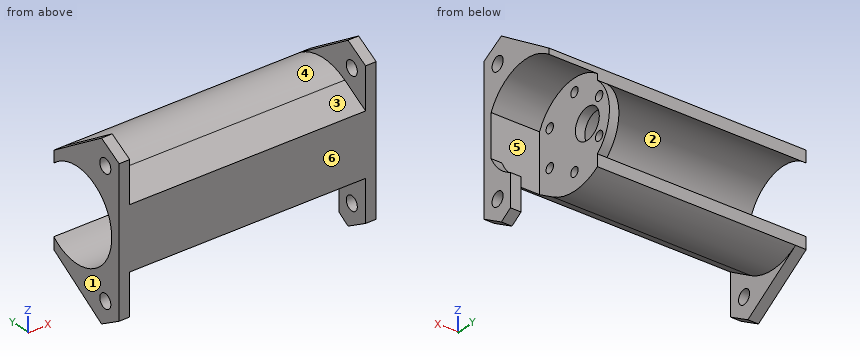
from build123d import *

# Parameters (mm, degrees)
SKETCH1_R           = 3
BOSS_EXTRUDE1_DEPTH = 54.5
CUT_EXTRUDE1_DEPTH  = 50
BOSS_EXTRUDE2_START = 34
SKETCH3_R           = 19
SKETCH3_R_2         = 6.5
SKETCH3_R_3         = 2
BOSS_EXTRUDE2_DEPTH = 4
CUT_EXTRUDE2_DEPTH  = 20.5
SKETCH5_W           = 31.652494028
SKETCH5_H           = 22.199486155
CUT_EXTRUDE3_DEPTH  = 16


# Read off the part's stored shape, not the designer's step: Cut-Extrude2
with BuildPart() as part:
    # Sketch1 → Boss-Extrude1 (new, symmetric)
    with BuildSketch(Plane(origin=(0, 0, 0), x_dir=(0, 0, -1), z_dir=(1, 0, 0))):
        with BuildLine():
            Line((26.267851073, -23), (0, -23))
            Line((0, -23), (-26.267851073, -23))
            Line((-26.267851073, -23), (-30.597978092, -23))
            Line((-30.597978092, -23), (-36.109878886, -13.453107779))
            Line((-36.109878886, -13.453107779), (-19.306734576, 12.5))
            Line((-19.306734576, 12.5), (-14.309088021, 12.5))
            ThreePointArc((-14.309088021, 12.5), (0, -19), (14.309088021, 12.5))
            Line((14.309088021, 12.5), (19.306734576, 12.5))
            Line((19.306734576, 12.5), (36.109878886, -13.453107779))
            Line((36.109878886, -13.453107779), (30.597978092, -23))
            Line((30.597978092, -23), (26.267851073, -23))
        make_face()
        with Locations((26.267851073, -15.5)):
            Circle(SKETCH1_R, mode=Mode.SUBTRACT)
        with Locations((-26.267851073, -15.5)):
            Circle(SKETCH1_R, mode=Mode.SUBTRACT)
    extrude(amount=BOSS_EXTRUDE1_DEPTH, both=True)

    # Sketch2 → Cut-Extrude1 (cut, symmetric)
    with BuildSketch(Plane(origin=(0, 0, 0), x_dir=(0, 0, -1), z_dir=(1, 0, 0))):
        with BuildLine():
            Line((19.808543432, -11.68852459), (13.089377665, -23))
            Line((13.089377665, -23), (30.597978092, -23))
            Line((30.597978092, -23), (36.109878886, -13.453107779))
            Line((36.109878886, -13.453107779), (19.306734576, 12.5))
            ThreePointArc((19.306734576, 12.5), (22.995052161, 0.477049386), (19.808543432, -11.68852459))
        make_face()
        with BuildLine():
            Line((-19.808543432, -11.68852459), (-13.089377665, -23))
            Line((-13.089377665, -23), (-30.597978092, -23))
            Line((-30.597978092, -23), (-36.109878886, -13.453107779))
            Line((-36.109878886, -13.453107779), (-19.306734576, 12.5))
            ThreePointArc((-19.306734576, 12.5), (-22.995052161, 0.477049386), (-19.808543432, -11.68852459))
        make_face()
    extrude(amount=CUT_EXTRUDE1_DEPTH, both=True, mode=Mode.SUBTRACT)

    # Sketch3 → Boss-Extrude2 (add)
    with BuildSketch(Plane(origin=(0, 0, 0), x_dir=(0, 0, -1), z_dir=(1, 0, 0)).offset(BOSS_EXTRUDE2_START)):
        Circle(SKETCH3_R)
        with Locations((0, 7)):
            Circle(SKETCH3_R_2, mode=Mode.SUBTRACT)
        with Locations((15.5, 0)):
            Circle(SKETCH3_R_3, mode=Mode.SUBTRACT)
        with Locations((7.75, -13.423393759)):
            Circle(SKETCH3_R_3, mode=Mode.SUBTRACT)
        with Locations((-7.75, -13.423393759)):
            Circle(SKETCH3_R_3, mode=Mode.SUBTRACT)
        with Locations((-15.5, 0)):
            Circle(SKETCH3_R_3, mode=Mode.SUBTRACT)
        with Locations((-7.75, 13.423393759)):
            Circle(SKETCH3_R_3, mode=Mode.SUBTRACT)
        with Locations((7.75, 13.423393759)):
            Circle(SKETCH3_R_3, mode=Mode.SUBTRACT)
    extrude(amount=-BOSS_EXTRUDE2_DEPTH)

    # Cut-Extrude2 outline → Cut-Extrude2 (cut)
    with BuildSketch(Plane(origin=(34, 0, 0), x_dir=(0, 0, -1), z_dir=(1, 0, 0))):
        with BuildLine():
            ThreePointArc((14.309088021, 12.5), (17.298843892, -7.858116823), (0, -19))
            Line((0, -19), (8.94427191, -19))
            ThreePointArc((8.94427191, -19), (15.012010115, -14.684670657), (19.192540727, -8.523284605))
            Line((19.192540727, -8.523284605), (32.918101974, -8.523284605))
            Line((32.918101974, -8.523284605), (19.306734576, 12.5))
            Line((19.306734576, 12.5), (14.309088021, 12.5))
        make_face()
        with BuildLine():
            ThreePointArc((-16.874537031, 12.5), (-20.364558031, -5.126868071), (-8.94427191, -19))
            Line((-8.94427191, -19), (0, -19))
            ThreePointArc((0, -19), (-17.298843892, -7.858116823), (-14.309088021, 12.5))
            Line((-14.309088021, 12.5), (-16.874537031, 12.5))
        make_face()
    extrude(amount=CUT_EXTRUDE2_DEPTH, mode=Mode.SUBTRACT)

    # Sketch5 → Cut-Extrude3 (cut)
    with BuildSketch(Plane(origin=(34, 0, 0), x_dir=(0, 0, -1), z_dir=(1, 0, 0))):
        with Locations((24.770518924, -7.900256922)):
            Rectangle(SKETCH5_W, SKETCH5_H)
    extrude(amount=CUT_EXTRUDE3_DEPTH, mode=Mode.SUBTRACT)


solid = part.part
Design review of the part built by this model. Coordinates are the model's own, in mm. Face numbers are marked on the shaded views. A direction names the side the tool comes from. Round coordinates to 2 decimals unless told otherwise and drop trailing zeros. Write each loop counter-clockwise with the first axis right and the second up, starting at its lowest first coordinate (ties: lowest second). Pieces come first, ordered by that corner, then holes. Notation, with made-up numbers: (-23, 52.25) -> (-8, 52.25) arc R22 cw to (-8, 83.25) -> close; hole circle Ø4 at (27, 65.5). An arc over 180 degrees is marked (long way). One line per question, with ' | ' between items.
(1) Machinability: for the marked faces 4, 5 and 6, which of the approach directions +Z, -Z, +X, -X, +Y, -Y give a long, thin tool a straight path to every point of the face, cutting with its end or side? Answer none if there is none.
Result sheet:
face 4: +Z | face 5: +Y | face 6: +Z, -Z, +X, -X, -Y
(2) Take a section at B-B, the plane y = 4.5. State the section outline as (x, z) points, and give its area (3 significant figures).
Result sheet:
outline: (-54.5, -24.49) -> (-50, -24.49) -> (-50, -22.56) -> (34, -22.56) -> (34, -6) -> (30, -6) -> (30, -18.46) -> (-54.5, -18.46) -> close; (-54.5, 18.46) -> (30, 18.46) -> (30, 6) -> (34, 6) -> (34, 20.51) -> (54.5, 20.51) -> (54.5, 24.49) -> (50, 24.49) -> (50, 22.56) -> (-50, 22.56) -> (-50, 24.49) -> (-54.5, 24.49) -> close | area: 893 mm2
(3) Take a section at A-A, the plane z = 15.5. State the section outline as (x, y) points, and give its area (3 significant figures).
Result sheet:
outline: (-54.5, -23) -> (-50, -23) -> (-50, -18.94) -> (50, -18.94) -> (50, -23) -> (54.5, -23) -> (54.5, -14.17) -> (34, -14.17) -> (34, -2) -> (30, -2) -> (30, -10.99) -> (-54.5, -10.99) -> close; (-54.5, 10.99) -> (30, 10.99) -> (30, 2) -> (34, 2) -> (34, 12.5) -> (-54.5, 12.5) -> close | area: 1,040 mm2
(4) Wall thickness on line 1 (Z direction, x = -25, y = -12.5); line 2 (X direction, y = -20.5, z = 22); line 3 (Z direction, x = 5, y = 0.5): over which ranges is each line inside the solid? List them lowest first. Write a range as [from, to].
Result sheet:
line 1: [-19.33, -14.31], [14.31, 19.33] | line 2: [-54.5, -50], [50, 54.5] | line 3: [-22.99, -18.99], [18.99, 22.99]
(5) Insertion check: P1, Ø2, axis at y = -0.5, z = 1, coming from the +X side; P2, Ø10, axis at x = -23, y = -1, coming from the -Z side; P3, Ø6.5, axis at y = -13.42, z = 7.75, coming from the -X side. Each pin has a flat end and moves straight along its axis. Give the tip position at first contact, or say it passes through.
Result sheet:
P1: x = 34 | P2: z = -23 | P3: x = 30
(6) Take a section at C-C, the plane x = -34. State the section outline as (y, z) points.
Result sheet:
outline: (-23, -13.09) -> (-11.69, -19.81) arc R23 ccw to (12.5, -19.31) -> (12.5, -14.31) arc R19 cw (long way) to (12.5, 14.31) -> (12.5, 19.31) arc R23 ccw to (-11.69, 19.81) -> (-23, 13.09) -> close
(7) Draft analysis for pull direction X (two halves, no side actions). For the marked faces 1, 2 and 3, state which applies: released by +X, released by -X, zero draft, split by the parting line, or undercut.
Result sheet:
face 1: released by -X | face 2: zero draft | face 3: undercut
(8) Take a section at D-D, the plane z = 26. State the section outline as (x, y) points.
Result sheet:
outline: (-54.5, -23) -> (-50, -23) -> (-50, -18.49) -> (-54.5, -18.49) -> close; (-54.5, -12.51) -> (-50, -12.51) -> (-50, 2.16) -> (-54.5, 2.16) -> close; (50, -23) -> (54.5, -23) -> (54.5, -18.49) -> (50, -18.49) -> close; (50, -12.51) -> (54.5, -12.51) -> (54.5, 2.16) -> (50, 2.16) -> close
